```python
from build123d import *

# Parameters (mm, degrees)
SKETCH_R        = 7.5
PAD_DEPTH       = 5
SKETCH001_R     = 5.4
PAD001_DEPTH    = 3
SKETCH002_R     = 7.5
PAD002_DEPTH    = 3
SKETCH003_R     = 5.4
PAD003_DEPTH    = 3
SKETCH004_R     = 7.5
PAD004_DEPTH    = 15
PAD005_DEPTH    = 5
PAD006_DEPTH    = 3
PAD007_DEPTH    = 5
SKETCH008_R     = 3.05
POCKET_DEPTH    = 34.001
CHAMFER_SIZE    = 2
CHAMFER001_SIZE = 2
CHAMFER002_SIZE = 2
CHAMFER003_SIZE = 2


with BuildPart() as part:
    # Sketch → Pad (new body)
    with BuildSketch(Plane.XY):
        Circle(SKETCH_R)
    extrude(amount=PAD_DEPTH)

    # Sketch001 (on Face3 of Pad) → Pad001 (join)
    with BuildSketch(Plane.XY.offset(5)):
        Circle(SKETCH001_R)
    extrude(amount=PAD001_DEPTH)

    # Sketch002 (on Face5 of Pad001) → Pad002 (join)
    with BuildSketch(Plane.XY.offset(8)):
        Circle(SKETCH002_R)
    extrude(amount=PAD002_DEPTH)

    # Sketch003 (on Face3 of Pad002) → Pad003 (join)
    with BuildSketch(Plane.XY.offset(11)):
        Circle(SKETCH003_R)
    extrude(amount=PAD003_DEPTH)

    # Sketch004 (on Face7 of Pad003) → Pad004 (join)
    with BuildSketch(Plane.XY.offset(14)):
        Circle(SKETCH004_R)
    extrude(amount=PAD004_DEPTH)

    # Sketch005 (on Face3 of Pad004) → Pad005 (join)
    with BuildSketch(Plane.XY.offset(29)):
        with BuildLine():
            ThreePointArc((-11.5, 11.5), (-23, 0), (-11.5, -11.5))
            Line((-11.5, -11.5), (11.5, -11.5))
            ThreePointArc((11.5, -11.5), (23, 0), (11.5, 11.5))
            Line((-11.5, 11.5), (11.5, 11.5))
        make_face()
    extrude(amount=PAD005_DEPTH)

    # Sketch006 (on Face4 of Pad005) → Pad006 (join)
    with BuildSketch(Plane(origin=(0, 0, 29), x_dir=(1, 0, 0), z_dir=(0, 0, -1))):
        with BuildLine():
            ThreePointArc((13.315217, -11.355835), (23, 0), (13.315217, 11.355835))
            ThreePointArc((13.315217, -11.355835), (17.5, 0), (13.315217, 11.355835))
        make_face()
        with BuildLine():
            ThreePointArc((-13.315217, 11.355835), (-23, 0), (-13.315217, -11.355835))
            ThreePointArc((-13.315217, 11.355835), (-17.5, 0), (-13.315217, -11.355835))
        make_face()
    extrude(amount=PAD006_DEPTH)

    # Sketch007 (on Face13 of Pad006) → Pad007 (join)
    with BuildSketch(Plane(origin=(0, 0, 26), x_dir=(1, 0, 0), z_dir=(0, 0, -1))):
        with BuildLine():
            ThreePointArc((-12, 11.489125), (-23, 0), (-12, -11.489125))
            Line((-12, 11.489125), (-12, -11.489125))
        make_face()
        with BuildLine():
            Line((12, 11.489125), (12, -11.489125))
            ThreePointArc((12, -11.489125), (23, 0), (12, 11.489125))
        make_face()
    extrude(amount=PAD007_DEPTH)

    # Sketch008 → Pocket (cut, through all)
    with BuildSketch(Plane.XY.offset(34)):
        Circle(SKETCH008_R)
    extrude(amount=-POCKET_DEPTH, mode=Mode.SUBTRACT)

    # Chamfer
    chamfer_edges = [part.edges().sort_by_distance(p)[0] for p in [
        (23, 0, 21),
    ]]
    chamfer(chamfer_edges, length=CHAMFER_SIZE)

    # Chamfer001
    chamfer001_edges = [part.edges().sort_by_distance(p)[0] for p in [
        (-23, 0, 21),
    ]]
    chamfer(chamfer001_edges, length=CHAMFER001_SIZE)

    # Chamfer002
    chamfer002_edges = [part.edges().sort_by_distance(p)[0] for p in [
        (-7.5, 0, 0),
    ]]
    chamfer(chamfer002_edges, length=CHAMFER002_SIZE)

    # Chamfer003
    chamfer003_edges = [part.edges().sort_by_distance(p)[0] for p in [
        (-23, 0, 34),
        (0, 11.5, 34),
        (0, -11.5, 34),
        (23, 0, 34),
        (-3.05, 0, 34),
    ]]
    chamfer(chamfer003_edges, length=CHAMFER003_SIZE)


solid = part.part
```
Geometry: final body of the model. Coordinates: model frame, mm. A direction names the side the tool comes from. Round coordinates to 2 decimals unless told otherwise and drop trailing zeros. Write each loop counter-clockwise with the first axis right and the second up, starting at its lowest first coordinate (ties: lowest second). Pieces come first, ordered by that corner, then holes. Notation, with made-up numbers: M -16.5,76 L 6.5,76 A14 ccw 6.5,100 Z; hole C -17,62 d4. An arc over 180 degrees is marked long. Answer in a Markdown table with one row per item. Add a question column.
(1) Draft query along Y for faces 6 (the face through (-7.493, 0.33, 21.395)), 7 (the face through (17.5, 0.2, 27.5)), 8 (the face through (3, -5, 14)). Return one class per face: pulls with the +Y half, pulls with the -Y half, needs draft (parallel to the pull), parting line crosses it, or undercut.
(2) Contact query for flat-ended pins moving along their axis: pin 1 (12 mm diameter, centred on x = -0.5, z = 18, fed in from +Y); pin 2 (8 mm diameter, centred on y = 2.5, z = 19.5, fed in from +X); pin 3 (1 mm diameter, centred on y = 3, z = 18.5, fed in from +X); pin 4 (7 mm diameter, centred on x = 0, y = 0, fed in from -Z). Output: stop coordinate, or through.
(3) Cut plane C-C, the plane x = -6.5. Give the number of separate pieces and of enclosed holes in the cut face, then the cut area to 3 significant figures.
(4) Cut plane B-B, the plane z = 16. Return the cut outline in (x, y).
(5) Ray query, L1, parallel to Y at x = 0, z = 24.5; L2, parallel to Z at x = -13, y = 6.75; L3, parallel to Z at x = -5, y = 8.5. Return the intervals inside material, ascending.
(6) Reachability of faces 1 (the face through (-7.493, 0.33, 9.479)), 2 (the face through (12, 0, 24)), 3 (the face through (0, 11.5, 30)), 4 (the face through (3, -5, 8)), 5 (the face through (-21.123, 0.212, 33.875)) from +Z, -Z, +X, -X, +Y, -Y: full face, straight path, thin tool, end or side. Return the list, or none.
Established:
| question | item | result |
|---|---|---|
| 1 | face 6 | parting line crosses it |
| 1 | face 7 | undercut |
| 1 | face 8 | needs draft |
| 2 | pin 1 | y = 7.5 |
| 2 | pin 2 | x = 22.99 |
| 2 | pin 3 | x = 7.07 |
| 2 | pin 4 | z = 0 |
| 3 | separate pieces | 3 |
| 3 | enclosed holes | 0 |
| 3 | area | 273 mm² |
| 4 | outline | C 0,0 d15; hole C 0,0 d6.1 |
| 5 | L1 | -7.5 to -3.05, 3.05 to 7.5 |
| 5 | L2 | 21 to 26, 29 to 34 |
| 5 | L3 | 29 to 34 |
| 6 | face 1 | -Z |
| 6 | face 2 | -Z, +Y, -Y |
| 6 | face 3 | +Z, -Z, +X, -X, +Y |
| 6 | face 4 | none |
| 6 | face 5 | +Z, -X |
